Could you check a few things on this drawing? It's one solid part, dimensions in mm from its lowest x, y, z. A direction names the side the tool comes from. Give positions to 0.01 mm unless a question says otherwise; leave off trailing zeros. Loops run counter-clockwise (first coordinate to the right, second up) from the corner with the lowest first, then second, coordinate; pieces in that order, holes last.
Q1. Suppose I cut it at C-C (z = 2.3). List the corners of the cut face in (x, y) for me.
Q2. Suppose I cut it at D-D (y = 1). List the corners of the cut face in (x, z) for me, and give its area (3 significant figures).
Q3. I need wall thicknesses on probe 1 along Z at (x, y) = (3.25, 3); probe 2 along Y at (x, z) = (9.5, 0.85) (1 decimal); probe 3 along X at (y, z) = (3.25, 1.6) (1 decimal). Which ranges of each line are inside material? Lowest first, please.
Q4. Thinking about a two-plate mould opening in Y: for the marked faces 3, 4 and 5, which applies, pulls with the +Y half, pulls with the -Y half, needs draft (parallel to the pull), parting line crosses it, or undercut?
Q5. For the marked faces 1 and 2, which set-ups out of +Z, -Z, +X, -X, +Y, -Y let a thin tool reach every point of the face, with its end or its side?
Q6. Suppose I cut it at B-B (x = 4). List the corners of the cut face in (y, z) for me (1 decimal).
Q7. Suppose I cut it at A-A (z = 3.2). List the corners of the cut face in (x, y) for me (1 decimal).
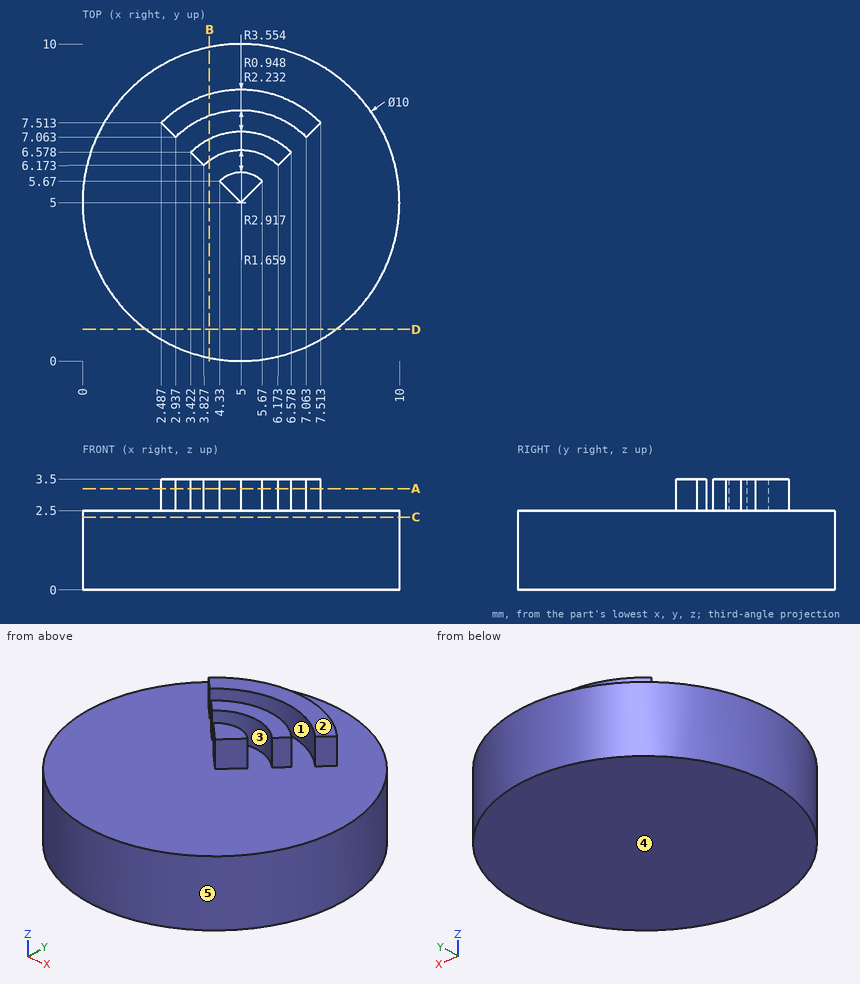
Solutions:
1. outline: circle Ø10 at (5, 5)
2. outline: (2, 0) - (8, 0) - (8, 2.5) - (2, 2.5) - close
2. area: 15.0 mm2
3. probe 1: z = 0 to 2.5
3. probe 2: y = 2.8 to 7.2
3. probe 3: x = 0.3 to 9.7
4. face 3: undercut
4. face 4: needs draft
4. face 5: parting line crosses it
5. face 1: +Z
5. face 2: +Z, +X, -X, +Y, -Y
6. outline: (0.1, 0) - (9.9, 0) - (9.9, 2.5) - (8.4, 2.5) - (8.4, 3.5) - (7.7, 3.5) - (7.7, 2.5) - (7, 2.5) - (7, 3.5) - (6.3, 3.5) - (6.3, 2.5) - (0.1, 2.5) - close
7. outline: (2.5, 7.5) - (2.9, 7.1) arc R2.9 cw to (7.1, 7.1) - (7.5, 7.5) arc R3.6 ccw to start; (3.4, 6.6) - (3.8, 6.2) arc R1.7 cw to (6.2, 6.2) - (6.6, 6.6) arc R2.2 ccw to start; (4.3, 5.7) - (5, 5) - (5.7, 5.7) arc R0.9 ccw to start
